Read the model definition and answer for the solid it produces. Units are mm, in the model's axes. Face numbers are marked on the shaded views. Round coordinates to 2 decimals unless told otherwise and drop trailing zeros. Order: outer loops, then holes, each group sorted by start corner. A loop starts at its lowest first (then second) coordinate and runs counter-clockwise, first axis right, second up.
Autodesk Inventor part; units mm, degrees
ref_plane "YZ Plane" through (0, 0, 0) normal (1, 0, 0) x (0, 1, 0)
ref_plane "XZ Plane" through (0, 0, 0) normal (0, 1, 0) x (-1, 0, 0)
ref_plane "XY Plane" through (0, 0, 0) normal (0, 0, 1) x (1, 0, 0)
sketch "Skizze1" plane through (0, 0, 0) normal (0, 1, 0) x (-1, 0, 0)
  circle A0 centre (0, 0) radius 1.8
  line L0 (0, 0) -> (-93.345, 0) construction
  line L1 (-93.345, 0) -> (-93.345, -92.71) construction
  line L2 (-93.345, -92.71) -> (0, -92.71) construction
  line L3 (0, -92.71) -> (0, 0) construction
  circle A1 centre (0, -92.71) radius 1.8
  circle A2 centre (-93.345, -92.71) radius 1.8
  circle A3 centre (-93.345, 0) radius 1.8
  circle A4 centre (-30.8, -92.71) radius 1.8
  circle A5 centre (-36.83, -92.71) radius 1.8
  circle A6 centre (-67.63, -92.71) radius 1.8
  line L4 (0, -63.81) -> (-93.345, -63.81) construction
  circle A7 centre (0, -63.81) radius 1.8
  circle A8 centre (-30.8, -63.81) radius 1.8
  circle A9 centre (-36.83, -63.81) radius 1.8
  circle A10 centre (-67.63, -63.81) radius 1.8
  line L5 (0.635, -95.885) -> (-93.98, -95.885) construction
  line L6 (-96.52, -93.345) -> (-96.52, 0.635) construction
  line L7 (-93.98, 3.175) -> (0.635, 3.175) construction
  line L8 (3.175, 0.635) -> (3.175, -93.345) construction
  arc A11 (0.635, -95.885) -> (3.175, -93.345) centre (0.635, -93.345) ccw construction
  arc A12 (-96.52, -93.345) -> (-93.98, -95.885) centre (-93.98, -93.345) ccw construction
  arc A13 (-93.98, 3.175) -> (-96.52, 0.635) centre (-93.98, 0.635) ccw construction
  arc A14 (3.175, 0.635) -> (0.635, 3.175) centre (0.635, 0.635) ccw construction
  line L9 (-93.98, -96.085) -> (0.635, -96.085)
  arc A15 (0.635, -96.085) -> (3.375, -93.345) centre (0.635, -93.345) ccw
  line L10 (3.375, -93.345) -> (3.375, 0.635)
  arc A16 (3.375, 0.635) -> (0.635, 3.375) centre (0.635, 0.635) ccw
  line L11 (0.635, 3.375) -> (-93.98, 3.375)
  arc A17 (-93.98, 3.375) -> (-96.72, 0.635) centre (-93.98, 0.635) ccw
  line L12 (-96.72, 0.635) -> (-96.72, -93.345)
  arc A18 (-96.72, -93.345) -> (-93.98, -96.085) centre (-93.98, -93.345) ccw
  line L13 (0.635, -97.085) -> (-93.98, -97.085)
  arc A19 (-97.72, -93.345) -> (-93.98, -97.085) centre (-93.98, -93.345) ccw
  line L14 (-97.72, -93.345) -> (-97.72, 0.635)
  arc A20 (-93.98, 4.375) -> (-97.72, 0.635) centre (-93.98, 0.635) ccw
  line L15 (-93.98, 4.375) -> (0.635, 4.375)
  arc A21 (4.375, 0.635) -> (0.635, 4.375) centre (0.635, 0.635) ccw
  line L16 (4.375, 0.635) -> (4.375, -93.345)
  arc A22 (0.635, -97.085) -> (4.375, -93.345) centre (0.635, -93.345) ccw
  line L17 (0.635, -95.285) -> (-93.98, -95.285)
  arc A23 (-95.92, -93.345) -> (-93.98, -95.285) centre (-93.98, -93.345) ccw
  line L18 (-95.92, -93.345) -> (-95.92, 0.635)
  arc A24 (-93.98, 2.575) -> (-95.92, 0.635) centre (-93.98, 0.635) ccw
  line L19 (-93.98, 2.575) -> (0.635, 2.575)
  arc A25 (2.575, 0.635) -> (0.635, 2.575) centre (0.635, 0.635) ccw
  line L20 (2.575, 0.635) -> (2.575, -93.345)
  arc A26 (0.635, -95.285) -> (2.575, -93.345) centre (0.635, -93.345) ccw
  line L21 (-3.8, -95.285) -> (-3.8, -90.91)
  line L22 (-1.8, -88.91) -> (2.575, -88.91)
  line L23 (-27, -95.285) -> (-27, -90.91)
  line L24 (-29, -88.91) -> (-38.63, -88.91)
  line L25 (-40.63, -90.91) -> (-40.63, -95.285)
  line L26 (-63.83, -95.285) -> (-63.83, -90.91)
  line L27 (-65.83, -88.91) -> (-69.43, -88.91)
  line L28 (-71.43, -90.91) -> (-71.43, -95.285)
  line L29 (-89.545, -95.285) -> (-89.545, -90.91)
  line L30 (-91.545, -88.91) -> (-95.92, -88.91)
  line L31 (-95.92, -3.8) -> (-91.545, -3.8)
  line L32 (-89.545, -1.8) -> (-89.545, 2.575)
  line L33 (2.575, -3.8) -> (-1.8, -3.8)
  line L34 (-3.8, -1.8) -> (-3.8, 2.575)
  line L35 (2.575, -67.61) -> (-1.8, -67.61)
  line L36 (-3.8, -65.61) -> (-3.8, -62.01)
  line L37 (-1.8, -60.01) -> (2.575, -60.01)
  line L38 (-29, -67.61) -> (-38.63, -67.61)
  line L39 (-40.63, -65.61) -> (-40.63, -62.01)
  line L40 (-38.63, -60.01) -> (-29, -60.01)
  line L41 (-27, -62.01) -> (-27, -65.61)
  line L42 (-65.83, -67.61) -> (-69.43, -67.61)
  line L43 (-71.43, -65.61) -> (-71.43, -62.01)
  line L44 (-69.43, -60.01) -> (-65.83, -60.01)
  line L45 (-63.83, -62.01) -> (-63.83, -65.61)
  arc A27 (-1.8, -88.91) -> (-3.8, -90.91) centre (-1.8, -90.91) ccw
  arc A28 (-27, -90.91) -> (-29, -88.91) centre (-29, -90.91) ccw
  arc A29 (-38.63, -88.91) -> (-40.63, -90.91) centre (-38.63, -90.91) ccw
  arc A30 (-63.83, -90.91) -> (-65.83, -88.91) centre (-65.83, -90.91) ccw
  arc A31 (-69.43, -88.91) -> (-71.43, -90.91) centre (-69.43, -90.91) ccw
  arc A32 (-89.545, -90.91) -> (-91.545, -88.91) centre (-91.545, -90.91) ccw
  arc A33 (-65.83, -67.61) -> (-63.83, -65.61) centre (-65.83, -65.61) ccw
  arc A34 (-71.43, -65.61) -> (-69.43, -67.61) centre (-69.43, -65.61) ccw
  arc A35 (-69.43, -60.01) -> (-71.43, -62.01) centre (-69.43, -62.01) ccw
  arc A36 (-63.83, -62.01) -> (-65.83, -60.01) centre (-65.83, -62.01) ccw
  arc A37 (-27, -62.01) -> (-29, -60.01) centre (-29, -62.01) ccw
  arc A38 (-29, -67.61) -> (-27, -65.61) centre (-29, -65.61) ccw
  arc A39 (-40.63, -65.61) -> (-38.63, -67.61) centre (-38.63, -65.61) ccw
  arc A40 (-38.63, -60.01) -> (-40.63, -62.01) centre (-38.63, -62.01) ccw
  arc A41 (-1.8, -60.01) -> (-3.8, -62.01) centre (-1.8, -62.01) ccw
  arc A42 (-3.8, -65.61) -> (-1.8, -67.61) centre (-1.8, -65.61) ccw
  arc A43 (-3.8, -1.8) -> (-1.8, -3.8) centre (-1.8, -1.8) ccw
  arc A44 (-91.545, -3.8) -> (-89.545, -1.8) centre (-91.545, -1.8) ccw
  point P0 (-27, -67.61)
  point P1 (-40.63, -60.01)
  point P2 (-27, -60.01)
  dimension "d0" = 3.6
  dimension "d1" = 3.6
  dimension "d2" = 3.6
  dimension "d3" = 3.6
  dimension "d4" = 93.345
  dimension "d5" = 92.71
  dimension "d6" = 3.6
  dimension "d7" = 3.6
  dimension "d8" = 3.6
  dimension "d10" = 3.6
  dimension "d11" = 3.6
  dimension "d12" = 3.6
  dimension "d13" = 3.6
  dimension "d14" = 28.9
  dimension "d15" = 30.8
  dimension "d16" = 6.03
  dimension "d17" = 30.8
  dimension "d18" = 30.8
  dimension "d19" = 6.03
  dimension "d20" = 30.8
  dimension "d21" = 3.175
  dimension "d22" = 2.54
  dimension "d23" = 0.2
  dimension "d24" = 1
  dimension "d29" = 0.8
  dimension "d32" = 3.8
  dimension "d33" = 3.8
  dimension "d35" = 3.8
  dimension "d36" = 3.8
  dimension "d37" = 3.8
  dimension "d38" = 3.8
  dimension "d39" = 3.8
  dimension "d40" = 3.8
  dimension "d41" = 3.8
  dimension "d42" = 3.8
  dimension "d43" = 3.8
  dimension "d44" = 3.8
  dimension "d45" = 2
extrude "Extrusion1" add sketch "Skizze1" against normal blind 1 contours A0 | A1 | A2 | A3 | A4 | A5 | A6 | A7 | A8 | A9 | A10 | A18 L12 A17 L11 A16 L10 A15 L9 | L13 A19 L14 A20 L15 A21 L16 A22 | L17 L21 A27 L22 L20 A26 | L17 L23 A28 L24 A29 L25 L26 A30 L27 A31 L28 L29 A32 L30 L18 L31 A44 L32 L19 L34 A43 L33 L20 L37 A41 L36 A42 L35 L22 A27 L21 | L17 L25 A29 L24 A28 L23 | L35 A42 L36 A41 L37 L20 | L17 L28 A31 L27 A30 L26 | L33 A43 L34 L19 A25 L20 | L17 A23 L18 L30 A32 L29 | L32 A44 L31 L18 A24 L19 | L38 A39 L39 A40 L40 A37 L41 A38 | L42 A34 L43 A35 L44 A36 L45 A33
extrude "Extrusion2" add sketch "Skizze1" along normal blind 6 contours L13 A19 L14 A20 L15 A21 L16 A22
extrude "Extrusion3" add sketch "Skizze1" along normal blind 4.4 contours A18 L12 A17 L11 A16 L10 A15 L9
extrude "Extrusion4" add sketch "Skizze1" along normal up to surface (4.4 mm away) contours L17 L21 A27 L22 L20 A26 | L17 L25 A29 L24 A28 L23 | L35 A42 L36 A41 L37 L20 | L17 L28 A31 L27 A30 L26 | L33 A43 L34 L19 A25 L20 | L17 A23 L18 L30 A32 L29 | L32 A44 L31 L18 A24 L19 | L38 A39 L39 A40 L40 A37 L41 A38 | L42 A34 L43 A35 L44 A36 L45 A33
chamfer "Fase1" distance 1 angle 45 8 edges at (97.72, -1, -46.355) (96.6246, -1, 3.2796) (46.6725, -1, 4.375) (-3.2796, -1, 3.2796) (-4.375, -1, -46.355) (-3.2796, -1, -95.9896) (46.6725, -1, -97.085) (96.6246, -1, -95.9896)
equation "\"d0\" = holeDim"
equation "\"d1\" = holeDim"
equation "\"d2\" = holeDim"
equation "\"d3\" = holeDim"
equation "\"d6\" = holeDim"
equation "\"d7\" = holeDim"
equation "\"d8\" = holeDim"
equation "\"d10\" = holeDim"
equation "\"d11\" = holeDim"
equation "\"d12\" = holeDim"
equation "\"d13\" = holeDim"
equation "\"d17\" = d15"
equation "\"d18\" = d15"
equation "\"d19\" = d16"
equation "\"d20\" = d15"
equation "\"d23\" = airGabWall"
equation "\"d24\" = topWallThick"
equation "\"d29\" = baseWallThick"
equation "\"d32\" = insertWallThick"
equation "\"d33\" = insertWallThick"
equation "\"d35\" = insertWallThick"
equation "\"d36\" = insertWallThick"
equation "\"d37\" = insertWallThick"
equation "\"d38\" = insertWallThick"
equation "\"d39\" = insertWallThick"
equation "\"d40\" = insertWallThick"
equation "\"d41\" = insertWallThick"
equation "\"d42\" = insertWallThick"
equation "\"d43\" = insertWallThick"
equation "\"d44\" = insertWallThick"
equation "\"d25\" = baseThick"
equation "\"d27\" = heightWall"
equation "\"d30\" = baseHeightWall"
equation "\"holeDim\" = 3.6"
equation "\"topWallThick\" = 1"
equation "\"airGabWall\" = 0.2"
equation "\"baseThick\" = 1"
equation "\"heightWall\" = heightInnerWall + pcbThick"
equation "\"baseWallThick\" = 0.8"
equation "\"pcbThick\" = 1.6"
equation "\"baseHeightWall\" = heightWall - pcbThick"
equation "\"heightInnerWall\" = 4.4"
properties part number "Housing_Bottom"
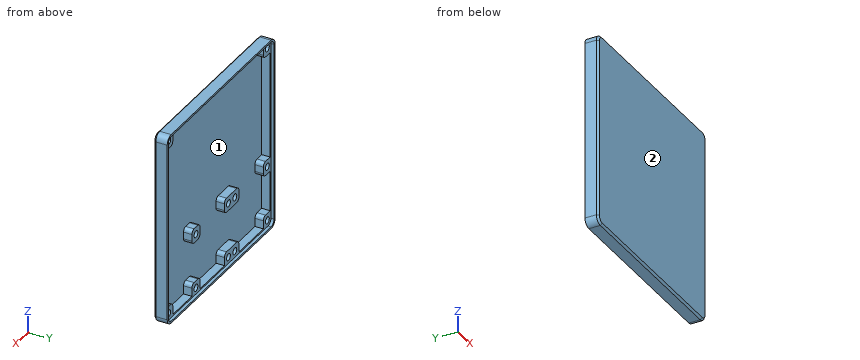
Q1. Straight lines are drawn through the part: probe 1 along Z at (x, y) = (67.63, 1.2) (3 decimals); probe 2 along Z at (x, y) = (0, 1.05) (3 decimals); probe 3 along Z at (x, y) = (57.5, 1.5) (3 decimals). For each, find the intervals that lie inside material, in ascending order.
Outcome:
probe 1: z = -97.085 to -94.51, -90.91 to -88.91, -67.61 to -65.61, -62.01 to -60.01, 2.575 to 4.375
probe 2: z = -97.085 to -94.51, -90.91 to -88.91, -67.61 to -65.61, -62.01 to -60.01, -3.8 to -1.8, 1.8 to 4.375
probe 3: z = -97.085 to -95.285, 2.575 to 4.375
Q2. A cutting plane is placed at A-A, the plane y = 1.5. Give the number of separate pieces and of enclosed holes in the cut face, plus the area to 3 significant figures.
Outcome:
separate pieces: 3
enclosed holes: 12
area: 1,090 mm2
Q3. A flat-ended cylindrical pin translates along its axis: pin 1 (1.1 mm diameter, centred on x = 0.5, z = -93, fed in from +Y). Find the tip coordinate at first contact, or state that the pin passes through.
Outcome:
pin 1: stops at y = 0
Q4. A cutting plane is placed at C-C, the plane z = -54. Give the vertices of the cut face in (x, y) (3 decimals).
Outcome:
outline: (-4.375, 0) - (-3.375, -1) - (96.72, -1) - (97.72, 0) - (97.72, 6) - (96.72, 6) - (96.72, 4.4) - (95.92, 4.4) - (95.92, 0) - (-2.575, 0) - (-2.575, 4.4) - (-3.375, 4.4) - (-3.375, 6) - (-4.375, 6) - close
Q5. For a pull along Z with two mould halves and no side action, classify the marked faces 1 and 2 as released by +Z, released by -Z, zero draft, split by the parting line, or undercut.
Outcome:
face 1: undercut
face 2: zero draft
Q6. A cutting plane is placed at B-B, the plane x = 36.83. Give the vertices of the cut face in (y, z) (3 decimals), plus the area to 3 significant figures.
Outcome:
outline: (-1, -96.085) - (0, -97.085) - (6, -97.085) - (6, -96.085) - (4.4, -96.085) - (4.4, -94.51) - (0, -94.51) - (0, -90.91) - (4.4, -90.91) - (4.4, -88.91) - (0, -88.91) - (0, -67.61) - (4.4, -67.61) - (4.4, -65.61) - (0, -65.61) - (0, -62.01) - (4.4, -62.01) - (4.4, -60.01) - (0, -60.01) - (0, 2.575) - (4.4, 2.575) - (4.4, 3.375) - (6, 3.375) - (6, 4.375) - (0, 4.375) - (-1, 3.375) - close
area: 149 mm2
